Source: CAD feature listing. Evaluate the final solid. Frame: model axes, mm. Coordinates: 2 decimals unless noted, no trailing zeros. Loops run counter-clockwise (first coordinate to the right, second up) from the corner with the lowest first, then second, coordinate; pieces in that order, holes last. Notation, with made-up numbers: (18, 56) -> (56, 56) arc R35 cw to (56, 93) -> close; hole circle Ø5 at (49, 39). An arc over 180 degrees is marked (long way). Answer as CSV lines item,"result".
from build123d import *

# Parameters (mm, degrees)
SKETCH_R  = 1.5
PAD_DEPTH = 3
FILLET_R  = 1


with BuildPart() as part:
    # Sketch → Pad (new body)
    with BuildSketch(Plane.XY):
        with BuildLine():
            Line((-16, 5), (16, 5))
            Line((16, 1.5), (16, 5))
            ThreePointArc((16, 1.5), (14.5, 0), (16, -1.5))
            Line((16, -1.5), (16, -5))
            Line((16, -5), (5, -5))
            Line((5, -5), (5, -35))
            Line((5, -35), (43, -35))
            Line((43, -35), (43, -45))
            Line((43, -45), (-5, -45))
            Line((-5, -45), (-5, -35))
            Line((-5, -35), (-5, -5))
            Line((-5, -5), (-16, -5))
            Line((-16, -5), (-16, -1.5))
            ThreePointArc((-16, -1.5), (-14.5, 0), (-16, 1.5))
            Line((-16, 5), (-16, 1.5))
        make_face()
        with Locations((-8, 0)):
            Circle(SKETCH_R, mode=Mode.SUBTRACT)
        Circle(SKETCH_R, mode=Mode.SUBTRACT)
        with Locations((8, 0)):
            Circle(SKETCH_R, mode=Mode.SUBTRACT)
        with Locations((0, -8)):
            Circle(SKETCH_R, mode=Mode.SUBTRACT)
        with Locations((0, -16)):
            Circle(SKETCH_R, mode=Mode.SUBTRACT)
        with Locations((0, -24)):
            Circle(SKETCH_R, mode=Mode.SUBTRACT)
        with Locations((0, -32)):
            Circle(SKETCH_R, mode=Mode.SUBTRACT)
        with Locations((0, -40)):
            Circle(SKETCH_R, mode=Mode.SUBTRACT)
        with Locations((8, -40)):
            Circle(SKETCH_R, mode=Mode.SUBTRACT)
        with Locations((16, -40)):
            Circle(SKETCH_R, mode=Mode.SUBTRACT)
        with Locations((24, -40)):
            Circle(SKETCH_R, mode=Mode.SUBTRACT)
        with Locations((32, -40)):
            Circle(SKETCH_R, mode=Mode.SUBTRACT)
        with Locations((40, -40)):
            Circle(SKETCH_R, mode=Mode.SUBTRACT)
    extrude(amount=PAD_DEPTH)

    # Fillet
    fillet_edges = [part.edges().sort_by_distance(p)[0] for p in [
        (-16, 5, 1.5),
        (-16, -5, 1.5),
        (16, 5, 1.5),
        (16, -5, 1.5),
        (43, -35, 1.5),
        (5, -35, 1.5),
        (43, -45, 1.5),
        (-5, -45, 1.5),
        (5, -5, 1.5),
        (-5, -5, 1.5),
    ]]
    fillet(fillet_edges, radius=FILLET_R)


solid = part.part
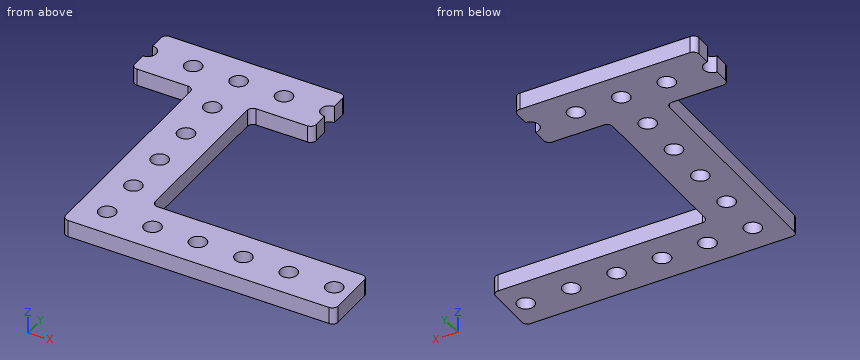
(1) Cut plane D-D (x = 24). Return the cut outline in (y, z), then the cut area to 3 significant figures.
Computed values:
outline,"(-45, 0) -> (-41.5, 0) -> (-41.5, 3) -> (-45, 3) -> close; (-38.5, 0) -> (-35, 0) -> (-35, 3) -> (-38.5, 3) -> close"
area,"21.0 mm^2"
(2) Pin query (flat end, axial travel): pin 1 Ø1.5 at (y, z) = (-20, 1) entering from -X; pin 2 Ø1.2 at (y, z) = (-3.5, 1) entering from +X; pin 3 Ø0.9 at (y, z) = (-16, 2) entering from +X. Return the tip coordinate at first contact, or that it passes through.
Computed values:
pin 1,"x = -5"
pin 2,"x = 16"
pin 3,"x = 5"
(3) Cut plane A-A (x = 8). Return the cut outline in (y, z), then the cut area to 3 significant figures.
Computed values:
outline,"(-45, 0) -> (-41.5, 0) -> (-41.5, 3) -> (-45, 3) -> close; (-38.5, 0) -> (-35, 0) -> (-35, 3) -> (-38.5, 3) -> close; (-5, 0) -> (-1.5, 0) -> (-1.5, 3) -> (-5, 3) -> close; (1.5, 0) -> (5, 0) -> (5, 3) -> (1.5, 3) -> close"
area,"42.0 mm^2"
(4) Material intervals for L1, parallel to Y at x = 8, z = 1.55; L2, parallel to Y at x = 6, z = 2.2; L3, parallel to Y at x = -13, z = 0.3, sorted ascending. Write a range as [from, to].
Computed values:
L1,"[-45, -41.5], [-38.5, -35], [-5, -1.5], [1.5, 5]"
L2,"[-45, -35], [-5, 5]"
L3,"[-5, 5]"
(5) Cut plane C-C (y = -40). Return the cut outline in (x, z).
Computed values:
outline,"(-5, 0) -> (-1.5, 0) -> (-1.5, 3) -> (-5, 3) -> close; (1.5, 0) -> (6.5, 0) -> (6.5, 3) -> (1.5, 3) -> close; (9.5, 0) -> (14.5, 0) -> (14.5, 3) -> (9.5, 3) -> close; (17.5, 0) -> (22.5, 0) -> (22.5, 3) -> (17.5, 3) -> close; (25.5, 0) -> (30.5, 0) -> (30.5, 3) -> (25.5, 3) -> close; (33.5, 0) -> (38.5, 0) -> (38.5, 3) -> (33.5, 3) -> close; (41.5, 0) -> (43, 0) -> (43, 3) -> (41.5, 3) -> close"
(6) Cut plane B-B (y = -24). Return the cut outline in (x, z), then the cut area to 3 significant figures.
Computed values:
outline,"(-5, 0) -> (-1.5, 0) -> (-1.5, 3) -> (-5, 3) -> close; (1.5, 0) -> (5, 0) -> (5, 3) -> (1.5, 3) -> close"
area,"21.0 mm^2"
